Model file for the job. Use its own axes, mm. A direction names the side the tool comes from. Give positions to 0.01 mm unless a question says otherwise; leave off trailing zeros. Write each loop counter-clockwise with the first axis right and the second up, starting at its lowest first coordinate (ties: lowest second). Pieces come first, ordered by that corner, then holes. Notation, with made-up numbers: (-27.75, 23.25) - (-8.75, 23.25) arc R19 ccw to (-8.75, 53.25) - close; hole circle Ø3 at (13, 17.25). An arc over 180 degrees is marked (long way). Use a Markdown table: item, result. Add a question column.
```python
from build123d import *

# Parameters (mm, degrees)
SKETCH1_R           = 45.85
SKETCH1_R_2         = 1.5635
SKETCH1_R_3         = 39.5
BOSS_EXTRUDE1_DEPTH = 4.7625
BOSS_EXTRUDE2_START = 4.7625
SKETCH1_4_R         = 45.85
SKETCH1_4_R_2       = 1.5635
SKETCH1_4_R_3       = 27.9
BOSS_EXTRUDE2_DEPTH = 4.7625
CUT_EXTRUDE2_DEPTH  = 4.7625
BOSS_EXTRUDE3_START = 4.7625
SKETCH3_R           = 45.85
SKETCH3_R_2         = 1.565
SKETCH3_R_3         = 3
SKETCH3_R_4         = 27.9
BOSS_EXTRUDE3_DEPTH = 4.7625
SKETCH6_R           = 1.46
CUT_EXTRUDE4_DEPTH  = 67.397120843


with BuildPart() as part:
    # Sketch1 → Boss-Extrude1 (new body)
    with BuildSketch(Plane(origin=(0, 0, 0), x_dir=(1, 0, 0), z_dir=(0, 1, 0))):
        with Locations(Location((0, 0, 0), (0, 0, 270))):
            Circle(SKETCH1_R)
        with Locations(Location((42.5, 0, 0), (0, 0, 270))):
            Circle(SKETCH1_R_2, mode=Mode.SUBTRACT)
        with Locations(Location((30.0520382, -30.0520382, 0), (0, 0, 270))):
            Circle(SKETCH1_R_2, mode=Mode.SUBTRACT)
        with Locations(Location((0, -42.5, 0), (0, 0, 270))):
            Circle(SKETCH1_R_2, mode=Mode.SUBTRACT)
        with Locations(Location((0, 0, 0), (0, 0, 270))):
            Circle(SKETCH1_R_3, mode=Mode.SUBTRACT)
        with Locations(Location((-30.0520382, -30.0520382, 0), (0, 0, 270))):
            Circle(SKETCH1_R_2, mode=Mode.SUBTRACT)
        with Locations(Location((-42.5, 0, 0), (0, 0, 270))):
            Circle(SKETCH1_R_2, mode=Mode.SUBTRACT)
        with Locations(Location((-30.0520382, 30.0520382, 0), (0, 0, 270))):
            Circle(SKETCH1_R_2, mode=Mode.SUBTRACT)
        with Locations(Location((0, 42.5, 0), (0, 0, 270))):
            Circle(SKETCH1_R_2, mode=Mode.SUBTRACT)
        with Locations(Location((30.0520382, 30.0520382, 0), (0, 0, 270))):
            Circle(SKETCH1_R_2, mode=Mode.SUBTRACT)
    extrude(amount=-BOSS_EXTRUDE1_DEPTH)

    # Sketch1_4 → Boss-Extrude2 (add)
    with BuildSketch(Plane(origin=(0, 0, 0), x_dir=(1, 0, 0), z_dir=(0, 1, 0)).offset(BOSS_EXTRUDE2_START)):
        with Locations(Location((0, 0, 0), (0, 0, 270))):
            Circle(SKETCH1_4_R)
        with Locations(Location((-30.0520382, -30.0520382, 0), (0, 0, 270))):
            Circle(SKETCH1_4_R_2, mode=Mode.SUBTRACT)
        with Locations(Location((0, -42.5, 0), (0, 0, 270))):
            Circle(SKETCH1_4_R_2, mode=Mode.SUBTRACT)
        with Locations(Location((30.0520382, -30.0520382, 0), (0, 0, 270))):
            Circle(SKETCH1_4_R_2, mode=Mode.SUBTRACT)
        with Locations(Location((-42.5, 0, 0), (0, 0, 270))):
            Circle(SKETCH1_4_R_2, mode=Mode.SUBTRACT)
        with Locations(Location((-30.0520382, 30.0520382, 0), (0, 0, 270))):
            Circle(SKETCH1_4_R_2, mode=Mode.SUBTRACT)
        with Locations(Location((42.5, 0, 0), (0, 0, 270))):
            Circle(SKETCH1_4_R_2, mode=Mode.SUBTRACT)
        with Locations(Location((0, 42.5, 0), (0, 0, 270))):
            Circle(SKETCH1_4_R_2, mode=Mode.SUBTRACT)
        with Locations(Location((30.0520382, 30.0520382, 0), (0, 0, 270))):
            Circle(SKETCH1_4_R_2, mode=Mode.SUBTRACT)
        with Locations(Location((0, 0, 0), (0, 0, 90))):
            Circle(SKETCH1_4_R_3, mode=Mode.SUBTRACT)
    extrude(amount=-BOSS_EXTRUDE2_DEPTH)

    # Sketch4 → Cut-Extrude2 (cut)
    with BuildSketch(Plane(origin=(0, 4.7625, 0), x_dir=(1, 0, 0), z_dir=(0, 1, 0))):
        Polygon((28.493192474, -27.3520382), (26.934346747, -30.0520382), (28.493192474, -32.7520382), (31.610883927, -32.7520382), (33.169729654, -30.0520382), (31.610883927, -27.3520382), align=None)
        Polygon((30.0520382, 33.169729654), (27.3520382, 31.610883927), (27.3520382, 28.493192474), (30.0520382, 26.934346747), (32.7520382, 28.493192474), (32.7520382, 31.610883927), align=None)
        Polygon((-27.3520382, -28.493192474), (-30.0520382, -26.934346747), (-32.7520382, -28.493192474), (-32.7520382, -31.610883927), (-30.0520382, -33.169729654), (-27.3520382, -31.610883927), align=None)
        Polygon((-28.493192474, 27.3520382), (-26.934346747, 30.0520382), (-28.493192474, 32.7520382), (-31.610883927, 32.7520382), (-33.169729654, 30.0520382), (-31.610883927, 27.3520382), align=None)
    extrude(amount=-CUT_EXTRUDE2_DEPTH, mode=Mode.SUBTRACT)

    # Sketch3 → Boss-Extrude3 (add)
    with BuildSketch(Plane(origin=(0, 4.7625, 0), x_dir=(1, 0, 0), z_dir=(0, 1, 0)).offset(BOSS_EXTRUDE3_START)):
        with Locations(Location((0, 0, 0), (0, 0, 270))):
            Circle(SKETCH3_R)
        with Locations(Location((-30.0520382, -30.0520382, 0), (0, 0, 90))):
            Circle(SKETCH3_R_2, mode=Mode.SUBTRACT)
        with Locations(Location((0, -42.5, 0), (0, 0, 90))):
            Circle(SKETCH3_R_3, mode=Mode.SUBTRACT)
        with Locations(Location((30.0520382, -30.0520382, 0), (0, 0, 90))):
            Circle(SKETCH3_R_2, mode=Mode.SUBTRACT)
        with Locations(Location((-42.5, 0, 0), (0, 0, 90))):
            Circle(SKETCH3_R_3, mode=Mode.SUBTRACT)
        with Locations(Location((-30.0520382, 30.0520382, 0), (0, 0, 90))):
            Circle(SKETCH3_R_2, mode=Mode.SUBTRACT)
        with Locations(Location((0, 0, 0), (0, 0, 90))):
            Circle(SKETCH3_R_4, mode=Mode.SUBTRACT)
        with Locations(Location((42.5, 0, 0), (0, 0, 90))):
            Circle(SKETCH3_R_3, mode=Mode.SUBTRACT)
        with Locations(Location((0, 42.5, 0), (0, 0, 90))):
            Circle(SKETCH3_R_3, mode=Mode.SUBTRACT)
        with Locations(Location((30.0520382, 30.0520382, 0), (0, 0, 90))):
            Circle(SKETCH3_R_2, mode=Mode.SUBTRACT)
    extrude(amount=-BOSS_EXTRUDE3_DEPTH)

    # Sketch6 → Cut-Extrude4 (cut, through all)
    with BuildSketch(Plane(origin=(0, 9.525, 0), x_dir=(1, 0, 0), z_dir=(0, 1, 0))):
        with Locations(Location((-40.188759664, 16.646729308, 0), (0, 0, 270))):
            Circle(SKETCH6_R)
        with Locations(Location((16.646729308, 40.188759664, 0), (0, 0, 270))):
            Circle(SKETCH6_R)
        with Locations(Location((-16.646729308, -40.188759664, 0), (0, 0, 270))):
            Circle(SKETCH6_R)
        with Locations(Location((40.188759664, -16.646729308, 0), (0, 0, 270))):
            Circle(SKETCH6_R)
    extrude(amount=-CUT_EXTRUDE4_DEPTH, mode=Mode.SUBTRACT)


solid = part.part
```
(1) Two-plate mould, pull along Z, no slides. Class faces 4 (the flat face through (38, -4.762, -14)), 5 (the flat face through (-27.725, 2.415, -28.683)): +Z half, -Z half, draft (parallel to the pull), parting line (faces both ways), or undercut.
(2) Band-saw the part on A-A (z = 0). Give the number of separate pieces and of enclosed holes in the cut face, then the cut area to 3 significant figures.
(3) Probe probe 1 along Z at (x, y) = (-41, 5.75); probe 2 along X at (y, z) = (1.75, 1); probe 3 along Z at (x, y) = (31, -3.5). List the from-to ranges inside material, lowest first. Write a range as [from, to].
(4) Flat gauge pins, fed straight in: pin 1 (3.5 mm diameter, centred on y = 3.5, z = 30.5, fed in from +X); pin 2 (1.9 mm diameter, centred on x = 30.05, z = -30.05, fed in from +Y); pin 3 (2 mm diameter, centred on y = -1, z = 30.5, fed in from -X); pin 4 (8 mm diameter, centred on x = -27.5, z = -8, fed in from -Y). Where does each tip first touch, or does it go through?
(5) Band-saw the part on C-C (z = -14). Write the cut outline in (x, y) (1 decimal).
(6) Which spindle directions (+Z, -Z, +X, -X, +Y, -Y) get a long thin tool onto all of the face, cutting with end or side? Do faces 1 (the flat face through (30, 2, 27.352)), 2 (the flat face through (27, 0, 8)), 3 (the flat face through (-1, 4.762, 44)). Say none if no direction does.
Model answer:
| question | item | result |
|---|---|---|
| 1 | face 4 | draft |
| 1 | face 5 | undercut |
| 2 | separate pieces | 4 |
| 2 | enclosed holes | 0 |
| 2 | area | 286 mm^2 |
| 3 | probe 1 | z = [-20.52, -17.86], [-15.43, -2.6], [2.6, 20.52] |
| 3 | probe 2 | x = [-45.84, -43.7], [-41.3, -27.88], [27.88, 41.3], [43.7, 45.84] |
| 3 | probe 3 | z = [-33.78, -31.3], [-28.81, -24.48], [24.48, 28.81], [31.3, 33.78] |
| 4 | pin 1 | stops at x = 35.72 |
| 4 | pin 2 | passes through |
| 4 | pin 3 | stops at x = -35.1 |
| 4 | pin 4 | stops at y = 0 |
| 5 | outline | (-43.7, -4.8) - (-36.9, -4.8) - (-36.9, 0) - (-24.1, 0) - (-24.1, 9.5) - (-43.7, 9.5) - close; (24.1, 0) - (36.9, 0) - (36.9, -4.8) - (43.7, -4.8) - (43.7, 9.5) - (24.1, 9.5) - close |
| 6 | face 1 | none |
| 6 | face 2 | -Y |
| 6 | face 3 | +Y |
